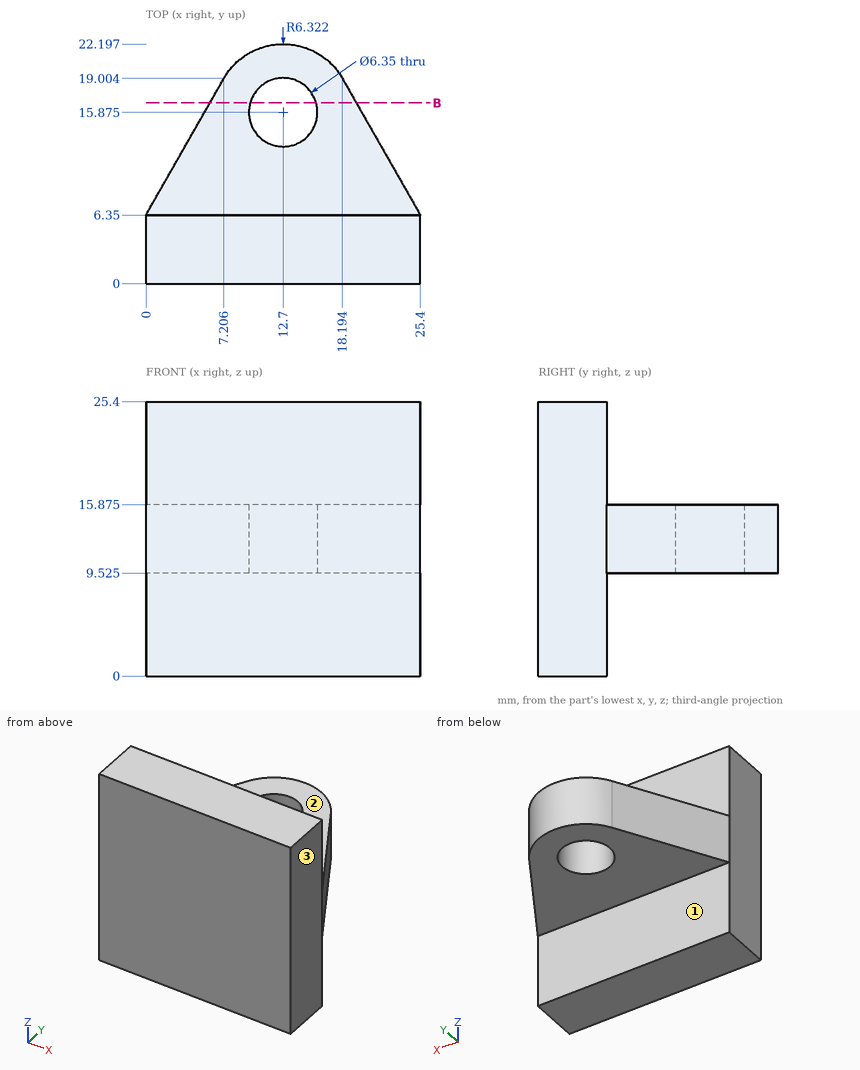
Here's the drawing with two shaded views (mm, measured from the low corner). I have some questions. A direction names the side the tool comes from. Round coordinates to 2 decimals unless told otherwise and drop trailing zeros. Order: outer loops, then holes, each group sorted by start corner. A loop starts at its lowest first (then second) coordinate and runs counter-clockwise, first axis right, second up. Notation, with made-up numbers: (1.5, 76) -> (16.5, 76) arc R20 cw to (16.5, 102) -> close; hole circle Ø1 at (30.25, -17.5). An arc over 180 degrees is marked (long way). Use a Markdown table: item, result. Add a question column.
(1) For pin 1 Ø4 at (x, y) = (4, 10) entering from -Z (3 decimals); pin 2 Ø10.5 at (x, z) = (8.5, 19.5) entering from +Y; pin 3 Ø5 at (x, y) = (15, 14) entering from +Z (3 decimals), each with a flat end and sliding along its axis, tell me the tip position at first contact or that it passes through.
(2) I need wall thicknesses on line 1 along Y through (x, z) = (12.7, 13); line 2 along Z through (x, y) = (7.5, 11.5) (1 decimal); line 3 along Y through (x, z) = (8, 1.75). Which ranges of each line are inside material? Lowest first, please.
(3) For the marked faces 1, 2 and 3, which set-ups out of +Z, -Z, +X, -X, +Y, -Y let a thin tool reach every point of the face, with its end or its side?
(4) Suppose I cut it at B-B, the plane y = 16.75. Please give me the cut outline in (x, z) (1 decimal), and give its area (3 significant figures).
Verdict:
| question | item | result |
|---|---|---|
| 1 | pin 1 | z = 9.525 |
| 1 | pin 2 | y = 22.18 |
| 1 | pin 3 | z = 15.875 |
| 2 | line 1 | 0 to 12.7, 19.05 to 22.2 |
| 2 | line 2 | 9.5 to 15.9 |
| 2 | line 3 | 0 to 6.35 |
| 3 | face 1 | -Z, +X, -X, +Y |
| 3 | face 2 | +Z, +X, -X, +Y |
| 3 | face 3 | +Z, -Z, +X, +Y, -Y |
| 4 | outline | (5.9, 9.5) -> (9.6, 9.5) -> (9.6, 15.9) -> (5.9, 15.9) -> close; (15.8, 9.5) -> (19.5, 9.5) -> (19.5, 15.9) -> (15.8, 15.9) -> close |
| 4 | area | 47.3 mm2 |
